Input: part model. Units: mm. Frame: model coordinates. Face numbers are marked on the shaded views. Coordinates: 2 decimals unless noted, no trailing zeros. Order: outer loops, then holes, each group sorted by start corner. A loop starts at its lowest first (then second) coordinate and runs counter-clockwise, first axis right, second up. Notation, with made-up numbers: (-2, -1) -> (42, -1) arc R27 ccw to (42, 23) -> close; hole circle Ø4 at (-5, 50.25). An arc over 180 degrees is marked (long way). One line per item, written item: value. Start each with the question number.
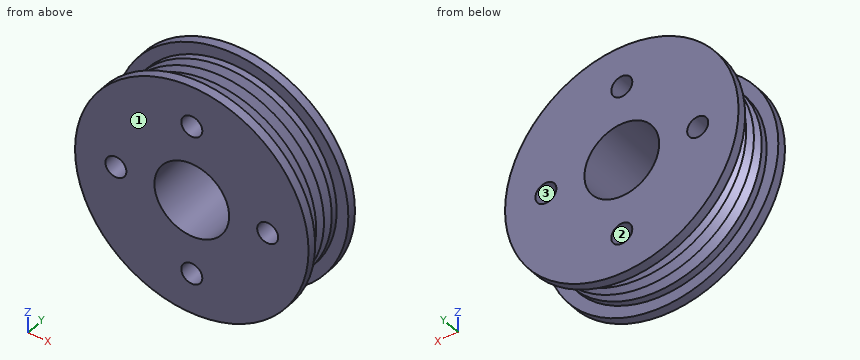
from build123d import *

# Parameters (mm, degrees)
ESBO_O2_R             = 2.25
ESBO_O2_R_2           = 8
CORTE_EXTRUS_O1_DEPTH = 14


with BuildPart() as part:
    # Esboço1 → Revolução1 (revolve)
    with BuildSketch(Plane.XY):
        Polygon((0, 7), (0, -7), (-25, -7), (-25, -5), (-22.5, -5), (-22.5, -3.51), (-20.7, -2.34), (-22.5, -1.17), (-20.7, 0), (-22.5, 1.17), (-20.7, 2.34), (-22.5, 3.51), (-22.5, 5), (-25, 5), (-25, 7), align=None)
    revolve(axis=Axis((0, 7, 0), (0, -1, 0)))

    # Esboço2 → Corte-extrusão1 (cut)
    with BuildSketch(Plane(origin=(0, 7, 0), x_dir=(1, 0, 0), z_dir=(0, 1, 0))):
        with Locations(Location((16.25, 0, 0), (0, 0, 180))):
            Circle(ESBO_O2_R)
        with Locations(Location((0, -16.25, 0), (0, 0, 180))):
            Circle(ESBO_O2_R)
        with Locations(Location((-16.25, 0, 0), (0, 0, 180))):
            Circle(ESBO_O2_R)
        with Locations(Location((0, 16.25, 0), (0, 0, 180))):
            Circle(ESBO_O2_R)
        with Locations(Location((0, 0, 0), (0, 0, 180))):
            Circle(ESBO_O2_R_2)
    extrude(amount=-CORTE_EXTRUS_O1_DEPTH, mode=Mode.SUBTRACT)


solid = part.part
1) Pin query (flat end, axial travel): pin 1 Ø3.5 at (x, z) = (0, -16.25) entering from -Y; pin 2 Ø1 at (y, z) = (0.5, -13.5) entering from +X; pin 3 Ø8 at (y, z) = (-5, 13.5) entering from -X; pin 4 Ø3 at (x, y) = (2.5, -0.5) entering from +Z. Return the tip coordinate at first contact, or that it passes through.
2) Section query A-A, the plane y = 4.25. Return the cut outline in (x, z).
3) Section query B-B, the plane x = 0. State how many separate pieces and enclosed holes the cut face has, plus the area to 3 significant figures.
4) Ray query, line 1 along Z through (x, y) = (0, -3.75); line 2 along Y through (x, z) = (-18, -15.5); line 3 along Y through (x, z) = (-2, -21.5). Return the intervals inside material, ascending. Write a range as from..to.
5) Mould query, pull axis Z, two halves, no side actions, for the marked faces 1, 2 and 3. Classes: +Z half, -Z half, draft (parallel to the pull), parting line (faces both ways), or undercut.
Entries:
1. pin 1: passes through
1. pin 2: stops at x = 17.74
1. pin 3: stops at x = -23.12
1. pin 4: stops at z = 22.47
2. outline: circle Ø45 at (0, 0); hole circle Ø4.5 at (-16.25, 0); hole circle Ø16 at (0, 0); hole circle Ø4.5 at (0, -16.25); hole circle Ø4.5 at (0, 16.25); hole circle Ø4.5 at (16.25, 0)
3. separate pieces: 4
3. enclosed holes: 0
3. area: 287 mm2
4. line 1: z = -22.5..-18.5, -14..-8, 8..14, 18.5..22.5
4. line 2: y = -7..-5, 5..7
4. line 3: y = -7..-2.92, -1.76..-0.58, 0.58..1.76, 2.92..7
5. face 1: draft
5. face 2: undercut
5. face 3: undercut
